from build123d import *

# Parameters (mm, degrees)
F0_W         = 64
F0_H         = 64
F1_DEPTH     = 6
F2_R         = 3
F3_DEPTH     = 2
F5_DEPTH     = 2
F7_T1_DEPTH  = 71.5
F7_T3_DEPTH  = 15.5
F7_T5_DEPTH  = 71.5
F7_S9_W      = 5
F7_S9_H      = 5
F7_T10_DEPTH = 5


# Not quite as in the source:
# - a fillet or chamfer that OpenCascade refuses, or shapes differently, is made with other operations: its cross-section is extruded or revolved along the edge and cut away or added
# - a feature of the source that left no trace in its solid (it failed there, or was rolled back) is left out


with BuildPart() as f1:
    # F0 (on Top) → F1 (new body)
    with BuildSketch(Plane.XY):
        with Locations((5.897675477, -1.6843453527)):
            Rectangle(F0_W, F0_H)
    extrude(amount=F1_DEPTH)

    # F2 (on Top) → F3 (cut)
    with BuildSketch(Plane.XY):
        with Locations((-16.102324523, 17.3156546473)):
            Circle(F2_R)
        with Locations((-6.1025285926, 17.3795400876)):
            Circle(F2_R)
    extrude(amount=F3_DEPTH, mode=Mode.SUBTRACT)

    # F4 (on face) → F5 (join)
    with BuildSketch(Plane.XY.offset(6)):
        Polygon((-23.111552, 27.8670135885), (-26.102324523, 27.8670135885), (-26.102324523, -33.6843453527), (-23.111552, -33.6843453527), (-23.111552, -30.7656601071), align=None)
        Polygon((-26.102324523, 30.3156546473), (-26.102324523, 27.8670135885), (-23.111552, 27.8670135885), (33.8885635138, 27.8670135885), (37.897675477, 27.8670135885), (37.897675477, 30.3156546473), align=None)
        Polygon((37.897675477, 27.8670135885), (33.8885635138, 27.8670135885), (33.8885635138, -30.7656601071), (37.897675477, -30.7656601071), (37.897675477, -12.6674966887), align=None)
        Polygon((33.8885635138, -30.7656601071), (-23.111552, -30.7656601071), (-23.111552, -33.6843453527), (37.897675477, -33.6843453527), (37.897675477, -30.7656601071), align=None)
    extrude(amount=F5_DEPTH)

    # F7: fillet of radius 5 on 3 edges, made by hand

    # F7_s2 → F7_t1 (cut)
    with BuildSketch(Plane.YZ.offset(-38.602324523)):
        with BuildLine():
            ThreePointArc((-33.6843453527, 3), (-32.2198792586, 6.5355339059), (-28.6843453527, 8))
            Line((-28.6843453527, 8), (-33.6843453527, 8))
            Line((-33.6843453527, 8), (-33.6843453527, 3))
        make_face()
    extrude(amount=F7_T1_DEPTH, mode=Mode.SUBTRACT)

    # F7_s4 → F7_t3 (cut)
    with BuildSketch(Plane.XY.offset(-12.5)):
        with BuildLine():
            ThreePointArc((32.897675477, -33.6843453527), (36.4332093829, -32.2198792586), (37.897675477, -28.6843453527))
            Line((37.897675477, -28.6843453527), (37.897675477, -33.6843453527))
            Line((37.897675477, -33.6843453527), (32.897675477, -33.6843453527))
        make_face()
    extrude(amount=F7_T3_DEPTH, mode=Mode.SUBTRACT)

    # F7_s6 → F7_t5 (cut)
    with BuildSketch(Plane.XZ.offset(-42.8156546473)):
        with BuildLine():
            ThreePointArc((37.897675477, 3), (36.4332093829, 6.5355339059), (32.897675477, 8))
            Line((32.897675477, 8), (37.897675477, 8))
            Line((37.897675477, 8), (37.897675477, 3))
        make_face()
    extrude(amount=F7_T5_DEPTH, mode=Mode.SUBTRACT)


with BuildPart() as f7_tool8:
    # F7_s9 → F7_t10 (new body)
    with BuildSketch(Plane.XZ.offset(28.6843453527)):
        with Locations((35.397675477, 5.5)):
            Rectangle(F7_S9_W, F7_S9_H)
    extrude(amount=F7_T10_DEPTH)

    # F7_s11 → F7_t12 (revolve, cut)
    with BuildSketch(Plane(origin=(32.897675477, -28.6843453527, 3), x_dir=(-0.7071067812, 0, -0.7071067812), z_dir=(-0.7071067812, 0, 0.7071067812))):
        with BuildLine():
            ThreePointArc((0, -5), (5, 0), (0, 5))
            Line((0, 5), (0, -5))
        make_face()
    revolve(axis=Axis((32.897675477, -28.6843453527, 3), (0, -1, 0)), mode=Mode.SUBTRACT)


with BuildPart() as f1_1:
    add(f1.part)

    # F7_t7: cut F7_tool8
    add(f7_tool8.part, mode=Mode.SUBTRACT)


solid = f1_1.part
Can you work these out from the model? Positions are in its coordinate system, mm. A direction names the side the tool comes from. Coordinates: 2 decimals unless noted, no trailing zeros. Loops run counter-clockwise (first coordinate to the right, second up) from the corner with the lowest first, then second, coordinate; pieces in that order, holes last. Notation, with made-up numbers: M 87,-15.75 L 110,-15.75 A9 ccw 110,-1.75 Z; hole C -6,41 d11. An arc over 180 degrees is marked long. Return JSON: item names as keys, results as strings. Group by question number.
Item 1: I'm going to push flat-ended pins straight in: pin 1 Ø4 at (y, z) = (-13, 7) entering from +X; pin 2 Ø2 at (x, y) = (21.5, -7.5) entering from +Z; pin 3 Ø2 at (x, z) = (1.5, 6.5) entering from -Y. Where does each tip first touch, or does it pass through?
Item 2: Imagine slicing it at B-B (x = 12.5). Please give me the cut outline in (y, z).
Item 3: If I drill on L1, parallel to Z at x = -8.5, y = -24; L2, parallel to X at y = 4, z = 6.5; L3, parallel to X at y = -19.5, z = 3.25, over which ranges is the centre line in solid material (lowest first)? Write a range as from..to.
Item 4: Imagine slicing it at D-D (y = 15.5). Please give me the cut outline in (x, z).
Item 5: Imagine slicing it at C-C (x = -17.5). Please give me the cut outline in (y, z).
Item 6: Imagine slicing it at A-A (y = -3). Please give me the cut outline in (x, z), and give its area (3 significant figures).
Item 7: On a 3-axis mill with a long thin cutter (end or side, diameter ignored), from which of +Z, -Z, +X, -X, +Y, -Y can I reach the whole of each face in a straight line? I mean faces 1 (the flat face through (6, -30.766, 7)), 2 (the cylindrical face through (-8.48, 15.55, 0.99)), 3 (the cylindrical face through (36.39, -32.26, 1.48)). Say none if no direction works.
Item 8: Thinking about a two-plate mould opening in X: for faces 4 (the flat face through (-26.102, -1, 4)), 5 (the cylindrical face through (36.47, 1.23, 6.5)), 6 (the flat face through (-23.112, -2, 7)), which applies, released by +X, released by -X, zero draft, split by the parting line, or undercut?
Verdict:
{
 "1": {"pin 1": "stops at x = 37.48", "pin 2": "stops at z = 6", "pin 3": "stops at y = -33.01"},
 "2": {"outline": "M -33.68,0 L 30.32,0 L 30.32,8 L 27.87,8 L 27.87,6 L -30.77,6 L -30.77,7.55 A5 ccw -33.68,3 Z"},
 "3": {"L1": "z = 0..6", "L2": "x = -26.1..-23.11, 33.89..36.47", "L3": "x = -26.1..37.89"},
 "4": {"outline": "M -26.1,0 L -18.49,0 L -18.49,2 L -13.71,2 L -13.71,0 L -8.44,0 L -8.44,2 L -3.76,2 L -3.76,0 L 37.9,0 L 37.9,3 A5 ccw 33.89,7.9 L 33.89,6 L -23.11,6 L -23.11,8 L -26.1,8 Z"},
 "5": {"outline": "M -33.68,0 L 14.66,0 L 14.66,2 L 19.97,2 L 19.97,0 L 30.32,0 L 30.32,8 L 27.87,8 L 27.87,6 L -30.77,6 L -30.77,7.55 A5 ccw -33.68,3 Z"},
 "6": {"outline": "M -26.1,0 L 37.9,0 L 37.9,3 A5 ccw 33.89,7.9 L 33.89,6 L -23.11,6 L -23.11,8 L -26.1,8 Z", "area": "393 mm^2"},
 "7": {"face 1": "+Z", "face 2": "-Z", "face 3": "+Z, -Z, +X, -Y"},
 "8": {"face 4": "released by -X", "face 5": "released by +X", "face 6": "undercut"}
}
